from build123d import *

# Parameters (mm, degrees)
SKETCH1_R           = 30
BOSS_EXTRUDE1_DEPTH = 110
SKETCH6_R           = 20
CUT_EXTRUDE2_DEPTH  = 100
SKETCH7_R           = 5
BOSS_EXTRUDE2_DEPTH = 35


with BuildPart() as part:
    # Sketch1 → Boss-Extrude1 (new body)
    with BuildSketch(Plane(origin=(0, 0, 0), x_dir=(1, 0, 0), z_dir=(0, 1, 0))):
        Circle(SKETCH1_R)
    extrude(amount=BOSS_EXTRUDE1_DEPTH)

    # Sketch5 → Revolve1 (revolve)
    with BuildSketch(Plane.XY):
        with BuildLine():
            Line((-30, 110), (0, 110))
            Line((0, 110), (30, 110))
            ThreePointArc((30, 110), (0, 140), (-30, 110))
        make_face()
    revolve(axis=Axis((-30, 110, 0), (1, 0, 0)))

    # Sketch6 → Cut-Extrude2 (cut)
    with BuildSketch(Plane.XZ):
        Circle(SKETCH6_R)
    extrude(amount=-CUT_EXTRUDE2_DEPTH, mode=Mode.SUBTRACT)

    # Sketch7 → Boss-Extrude2 (add)
    with BuildSketch(Plane(origin=(0, 0, 0), x_dir=(0, 0, -1), z_dir=(1, 0, 0))):
        with Locations((0, 110)):
            Circle(SKETCH7_R)
    boss_extrude2 = extrude(amount=BOSS_EXTRUDE2_DEPTH)

    # Mirror1: Boss-Extrude2 across plane
    add(boss_extrude2.mirror(Plane(origin=(0, 0, 0), x_dir=(0, 0, 1), z_dir=(1, 0, 0))))


solid = part.part
Source: CAD feature listing. Evaluate the final solid. Frame: model axes, mm. A direction names the side the tool comes from. Round coordinates to 2 decimals unless told otherwise and drop trailing zeros. Order: outer loops, then holes, each group sorted by start corner. A loop starts at its lowest first (then second) coordinate and runs counter-clockwise, first axis right, second up. Notation, with made-up numbers: (51.25, 47) -> (92.25, 47) arc R18 ccw to (92.25, 51) -> close; hole circle Ø6 at (11, 58). An arc over 180 degrees is marked (long way). Answer as CSV lines item,"result".
Item 1: Reachability of faces 1 (the face through (6, 0, 20)), 2 (the face through (-32.252, 114.957, 0.651)), 3 (the face through (-4.336, 49.3, -19.524)), 4 (the face through (32.252, 114.957, 0.651)) from +Z, -Z, +X, -X, +Y, -Y: full face, straight path, thin tool, end or side. Return the list, or none.
A:
face 1,"+Z, -Z, +X, -X, -Y"
face 2,"-X"
face 3,"-Y"
face 4,"+X"
Item 2: Section B-B, the plane z = 0. Return loops of the section in (x, y).
A:
outline,"(-35, 105) -> (-30, 105) -> (-30, 0) -> (-20, 0) -> (-20, 100) -> (20, 100) -> (20, 0) -> (30, 0) -> (30, 105) -> (35, 105) -> (35, 115) -> (29.58, 115) arc R30 ccw to (-29.58, 115) -> (-35, 115) -> close"
Item 3: Line query: L1, parallel to Z at x = 0, y = 66.5; L2, parallel to X at y = 42.5, z = 5; L3, parallel to Z at x = 13, y = 16.5. Output: solid intervals per line, ascending.
A:
L1,"-30 to -20, 20 to 30"
L2,"-29.58 to -19.36, 19.36 to 29.58"
L3,"-27.04 to -15.2, 15.2 to 27.04"
Item 4: Pin query (flat end, axial travel): pin 1 Ø2 at (x, z) = (6.5, -22) entering from +Y; pin 2 Ø12 at (y, z) = (114.5, 12.5) entering from +X; pin 3 Ø1 at (y, z) = (85.5, -13) entering from +X. Return the tip coordinate at first contact, or that it passes through.
A:
pin 1,"y = 130.46"
pin 2,"x = 29.1"
pin 3,"x = 27.27"
Item 5: Section A-A, the plane x = 0. Return loops of the section in (y, z), plus the area to 3 significant figures.
A:
outline,"(0, -30) -> (110, -30) arc R30 ccw to (110, 30) -> (0, 30) -> (0, 20) -> (100, 20) -> (100, -20) -> (0, -20) -> close"
area,"4,010 mm²"
Item 6: Section C-C, the plane y = 93.5. Return loops of the section in (x, z).
A:
outline,"circle Ø60 at (0, 0); hole circle Ø40 at (0, 0)"
Item 7: Section D-D, the plane y = 126. Return loops of the section in (x, z).
A:
outline,"circle Ø50.75 at (0, 0)"
Item 8: Pull-direction query (X, two-part tool) for faces 5 (the face through (35, 110, 0)), 6 (the face through (0, 100, 0)), 7 (the face through (-35, 110, 0)); classes: pulls with the +X half, pulls with the -X half, needs draft (parallel to the pull), parting line crosses it, or undercut.
A:
face 5,"pulls with the +X half"
face 6,"undercut"
face 7,"pulls with the -X half"
